Job drawing, mm, ordinate dimensions from the low corner. One solid piece. Give positions to 0.01 mm unless a question says otherwise; leave off trailing zeros. Write each loop counter-clockwise with the first axis right and the second up, starting at its lowest first coordinate (ties: lowest second). Pieces come first, ordered by that corner, then holes. Notation, with made-up numbers: (43.25, 74) - (74.25, 74) arc R4 cw to (74.25, 81) - close; hole circle Ø8 at (-35, 5.5). An arc over 180 degrees is marked (long way). Answer in a Markdown table with one row per item. Add a question column.
1. Probe line 1 along Y through (x, z) = (20, 2.25); line 2 along Y through (x, z) = (21, 1.35); line 3 along Y through (x, z) = (33.5, 1.7). List the from-to ranges inside material, lowest first.
2. Pull direction X, two halves, no side cores. Call the marked faces 1, 2 and 3: released by +X, released by -X, zero draft, split by the parting line, or undercut.
3. Drop a flat-ended pin along its axis: pin 1 Ø10 at (x, y) = (7.5, 35) entering from +Z. Give the stop position or say it passes through.
4. Band-saw the part on D-D on y = 20. Write the cut outline in (x, z), plus the area to 3 significant figures.
5. Band-saw the part on B-B on x = 26. Write the cut outline in (y, z).
6. Band-saw the part on A-A on y = 10. Write the cut outline in (x, z).
7. Band-saw the part on C-C on z = 4.65. State how many separate pieces and enclosed holes the cut face has, plus the area to 3 significant figures.
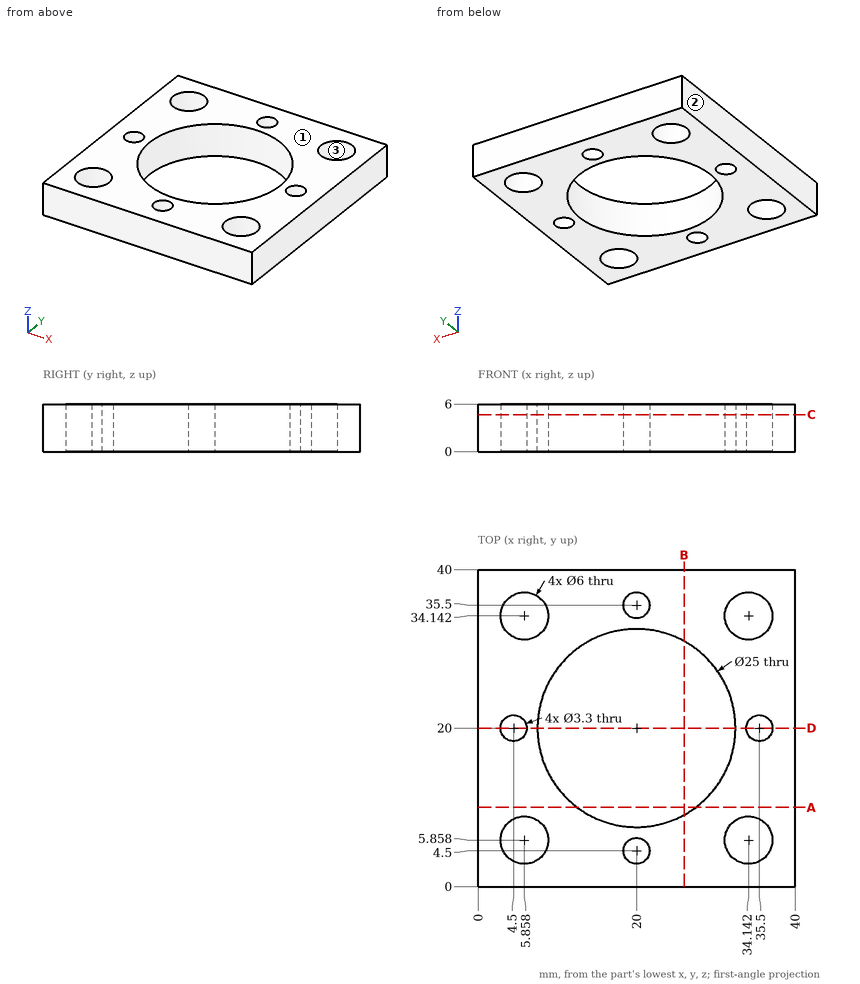
Values:
| question | item | result |
|---|---|---|
| 1 | line 1 | y = 0 to 2.85, 6.15 to 7.5, 32.5 to 33.85, 37.15 to 40 |
| 1 | line 2 | y = 0 to 3.19, 5.81 to 7.54, 32.46 to 34.19, 36.81 to 40 |
| 1 | line 3 | y = 0 to 2.93, 8.79 to 31.21, 37.07 to 40 |
| 2 | face 1 | zero draft |
| 2 | face 2 | released by -X |
| 2 | face 3 | undercut |
| 3 | pin 1 | stops at z = 6 |
| 4 | outline | (0, 0) - (2.85, 0) - (2.85, 6) - (0, 6) - close; (6.15, 0) - (7.5, 0) - (7.5, 6) - (6.15, 6) - close; (32.5, 0) - (33.85, 0) - (33.85, 6) - (32.5, 6) - close; (37.15, 0) - (40, 0) - (40, 6) - (37.15, 6) - close |
| 4 | area | 50.4 mm² |
| 5 | outline | (0, 0) - (9.03, 0) - (9.03, 6) - (0, 6) - close; (30.97, 0) - (40, 0) - (40, 6) - (30.97, 6) - close |
| 6 | outline | (0, 0) - (12.5, 0) - (12.5, 6) - (0, 6) - close; (27.5, 0) - (40, 0) - (40, 6) - (27.5, 6) - close |
| 7 | separate pieces | 1 |
| 7 | enclosed holes | 9 |
| 7 | area | 962 mm² |
